from build123d import *

# Parameters (mm, degrees)
SKETCH_R        = 30
PAD_DEPTH       = 70
SKETCH002_W     = 20.1
SKETCH002_H     = 20.1
POCKET_DEPTH    = 100
POCKET001_DEPTH = 100
FILLET_R        = 3


with BuildPart() as part:
    # Sketch → Pad (new body)
    with BuildSketch(Plane.XY):
        with BuildLine():
            ThreePointArc((19.899749, 30), (-36, 0), (19.899749, -30))
            Line((64, -30), (19.899749, -30))
            Line((64, 30), (64, -30))
            Line((19.899749, 30), (64, 30))
        make_face()
        Circle(SKETCH_R, mode=Mode.SUBTRACT)
    extrude(amount=PAD_DEPTH)

    # Sketch002 (on Face2 of Pad) → Pocket (cut)
    with BuildSketch(Plane.XZ.offset(30)):
        with Locations((42.05, 50.05)):
            Rectangle(SKETCH002_W, SKETCH002_H)
    extrude(amount=-POCKET_DEPTH, mode=Mode.SUBTRACT)

    # Sketch003 (on Face3 of Pocket) → Pocket001 (cut)
    with BuildSketch(Plane.XZ.offset(30)):
        Polygon((66, 30), (32, 0), (66, 0), align=None)
    extrude(amount=-POCKET001_DEPTH, mode=Mode.SUBTRACT)

    # Fillet
    fillet_edges = [part.edges().sort_by_distance(p)[0] for p in [
        (64, -30, 49.117647),
        (64, 30, 49.117647),
        (64, 0, 70),
        (64, 0, 28.235294),
        (48, 30, 14.117647),
        (48, -30, 14.117647),
        (41.949874, -30, 70),
        (41.949874, 30, 70),
    ]]
    fillet(fillet_edges, radius=FILLET_R)


solid = part.part
Design review of the part built by this model. Coordinates are the model's own, in mm. A direction names the side the tool comes from. Coordinates: 2 decimals unless noted, no trailing zeros. Order: outer loops, then holes, each group sorted by start corner. A loop starts at its lowest first (then second) coordinate and runs counter-clockwise, first axis right, second up.
Item 1: Take a section at C-C, the plane x = 0. Write out the cut boundary in (y, z), then the cut area to 3 significant figures.
Item 2: For pin 1 Ø12.5 at (x, z) = (33, 47) entering from +Y; pin 2 Ø10 at (x, y) = (38.5, -11.5) entering from -Z; pin 3 Ø3 at (x, z) = (14.5, 47.5) entering from +Y; pin 4 Ø12 at (x, y) = (-18.5, -20) entering from +Z, all flat-tipped, find the tip position at first contact; note any pin that passes through.
Item 3: The part is to be moulded in two halves that separate along Z. For faces 1 (the cylindrical face through (-29.97, 1.32, 34.51)), 2 (the cylindrical face through (45.39, -29.14, 13.01)), 3 (the flat face through (42, 0, 60.1)), say which applies: pulls with the +Z half, pulls with the -Z half, needs draft (parallel to the pull), parting line crosses it, or undercut.
Item 4: For faces 4 (the cylindrical face through (40.74, 29.14, 69.1)), 5 (the flat face through (42, 0, 40)), 6 (the cylindrical face through (40.16, -29.14, 69.1)), 7 (the flat face through (36, -30, 33)), list the 3-axis set-ups (+Z, -Z, +X, -X, +Y, -Y) from which the entire face can be reached by the end or side of a thin tool; tool diameter is ignored.
Item 5: Take a section at A-A, the plane z = 58.5. Write out the cut boundary in (x, y), then the cut area to 3 significant figures.
Item 6: For line 1 (Y direction, x = 0, z = 30); line 2 (Y direction, x = 59, z = 51.5); line 3 (Y direction, x = -2.5, z = 61), list the stretches that pass through material, from the lowest coordinate up.
Item 7: Take a section at B-B, the plane y = 0. Write out the cut boundary in (x, z).
Item 8: Take a section at D-D, the plane z = 38. Write out the cut boundary in (x, y).
The answers:
1. outline: (-36, 0) - (-30, 0) - (-30, 70) - (-36, 70) - close; (30, 0) - (36, 0) - (36, 70) - (30, 70) - close
1. area: 840 mm2
2. pin 1: stops at y = 30
2. pin 2: stops at z = 1.32
2. pin 3: stops at y = 33.57
2. pin 4: stops at z = 70
3. face 1: needs draft
3. face 2: pulls with the -Z half
3. face 3: undercut
4. face 4: +Z, +X, +Y
4. face 5: +Y, -Y
4. face 6: +Z, +X, -Y
4. face 7: +Z, -Z, +X, -Y
5. outline: (19.9, -30) - (32, -30) - (32, 30) - (19.9, 30) arc R36 ccw (long way) to start; (52.1, -30) - (61, -30) arc R3 ccw to (64, -27) - (64, 27) arc R3 ccw to (61, 30) - (52.1, 30) - close; hole circle Ø60 at (0, 0)
5. area: 2,000 mm2
6. line 1: y = -36 to -30, 30 to 36
6. line 2: y = -30 to 30
6. line 3: y = -35.91 to -29.9, 29.9 to 35.91
7. outline: (-36, 0) - (-30, 0) - (-30, 70) - (-36, 70) - close; (30, 0) - (32, 0) - (62.98, 27.34) arc R3 ccw to (64, 29.59) - (64, 67) arc R3 ccw to (61, 70) - (30, 70) - close; hole (32, 40) - (52.1, 40) - (52.1, 60.1) - (32, 60.1) - close
8. outline: (19.9, -30) - (61, -30) arc R3 ccw to (64, -27) - (64, 27) arc R3 ccw to (61, 30) - (19.9, 30) arc R36 ccw (long way) to start; hole circle Ø60 at (0, 0)
